For this review, take the finished solid that the model builds, in its own axes (mm). Face numbers are marked on the shaded views. A direction names the side the tool comes from. Round coordinates to 2 decimals unless told otherwise and drop trailing zeros. Loops run counter-clockwise (first coordinate to the right, second up) from the corner with the lowest first, then second, coordinate; pieces in that order, holes last. Notation, with made-up numbers: (23.25, -3.75) -> (55.25, -3.75) arc R26 ccw to (55.25, 34.25) -> close; hole circle Ø5 at (87.5, 68.5). An arc over 180 degrees is marked (long way). One line per question, with ' | ' between items. Start each with the question number.
1. Consider section A-A (y = 2). Write out the cut boundary in (x, z).
2. For the marked faces 4 and 5, list the 3-axis set-ups (+Z, -Z, +X, -X, +Y, -Y) from which the entire face can be reached by the end or side of a thin tool; tool diameter is ignored.
3. Consider section D-D (y = 6.5). Write out the cut boundary in (x, z).
4. Consider section C-C (z = 0.25). Write out the cut boundary in (x, y).
5. For pin 1 Ø1.2 at (x, y) = (26, 1.5) entering from -Z; pin 2 Ø1.6 at (y, z) = (7, -11) entering from +X; pin 3 Ø1.2 at (x, y) = (26, 1) entering from +Z, all flat-tipped, find the tip position at first contact; note any pin that passes through.
6. Wall thickness on line 1 along X through (y, z) = (8.5, 7.25); line 2 along Z through (x, y) = (3, 7.5): over which ranges is each line inside the solid? List them lowest first.
7. Consider section B-B (x = 2). Write out the cut boundary in (y, z), and give its area (3 significant figures).
8. Draft analysis for pull direction X (two halves, no side actions). For the marked faces 1, 2 and 3, state which applies: pulls with the +X half, pulls with the -X half, needs draft (parallel to the pull), parting line crosses it, or undercut.
```python
from build123d import *

# Parameters (mm, degrees)
SKETCH_1_W          = 50.5
SKETCH_1_H          = 23.5
EXTRUDE_1_DEPTH     = 12.2
SKETCH_2_W          = 7
SKETCH_2_H          = 4
EXTRUDE_2_DEPTH     = 1.5
SKETCH_3_W          = 18
SKETCH_3_H          = 8
CUT_EXTRUDE_1_DEPTH = 1.5


with BuildPart() as part:
    # Эскиз1 → Бобышка-Вытянуть1 (new body)
    with BuildSketch(Plane(origin=(0, 0, 0), x_dir=(1, 0, 0), z_dir=(0, 1, 0))):
        Rectangle(SKETCH_1_W, SKETCH_1_H)
    extrude(amount=EXTRUDE_1_DEPTH)

    # Эскиз2 → Бобышка-Вытянуть2 (add)
    with BuildSketch(Plane(origin=(25.25, 0, 0), x_dir=(0, 0, -1), z_dir=(1, 0, 0))):
        with Locations((0, 2)):
            Rectangle(SKETCH_2_W, SKETCH_2_H)
    extrude(amount=EXTRUDE_2_DEPTH)

    # Эскиз3 → Вырез-Вытянуть1 (cut)
    with BuildSketch(Plane.XY.offset(11.75)):
        with Locations((0, 8.2)):
            Rectangle(SKETCH_3_W, SKETCH_3_H)
    cut_extrude_1 = extrude(amount=-CUT_EXTRUDE_1_DEPTH, mode=Mode.SUBTRACT)

    # Зеркальное отражение1: Вырез-Вытянуть1 across plane
    add(cut_extrude_1.mirror(Plane.XY), mode=Mode.SUBTRACT)


solid = part.part
```
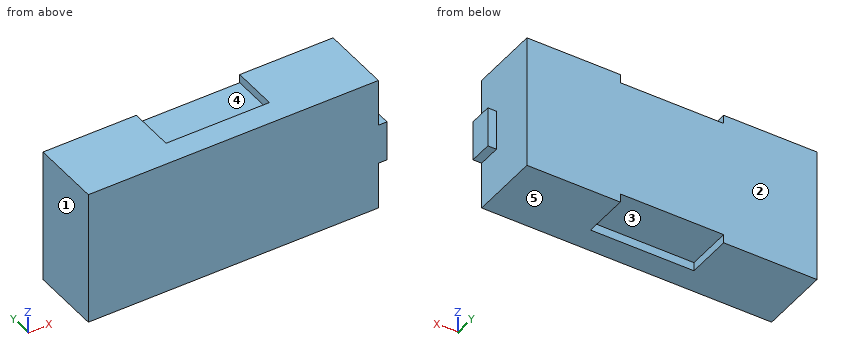
Answer block:
1) outline: (-25.25, -11.75) -> (25.25, -11.75) -> (25.25, -3.5) -> (26.75, -3.5) -> (26.75, 3.5) -> (25.25, 3.5) -> (25.25, 11.75) -> (-25.25, 11.75) -> close
2) face 4: +Z, +Y | face 5: -Z, +X, -X, +Y, -Y
3) outline: (-25.25, -11.75) -> (-9, -11.75) -> (-9, -10.25) -> (9, -10.25) -> (9, -11.75) -> (25.25, -11.75) -> (25.25, 11.75) -> (9, 11.75) -> (9, 10.25) -> (-9, 10.25) -> (-9, 11.75) -> (-25.25, 11.75) -> close
4) outline: (-25.25, 0) -> (26.75, 0) -> (26.75, 4) -> (25.25, 4) -> (25.25, 12.2) -> (-25.25, 12.2) -> close
5) pin 1: stops at z = -3.5 | pin 2: stops at x = 25.25 | pin 3: stops at z = 3.5
6) line 1: x = -25.25 to 25.25 | line 2: z = -10.25 to 10.25
7) outline: (0, -11.75) -> (4.2, -11.75) -> (4.2, -10.25) -> (12.2, -10.25) -> (12.2, 10.25) -> (4.2, 10.25) -> (4.2, 11.75) -> (0, 11.75) -> close | area: 263 mm2
8) face 1: pulls with the -X half | face 2: needs draft | face 3: undercut
